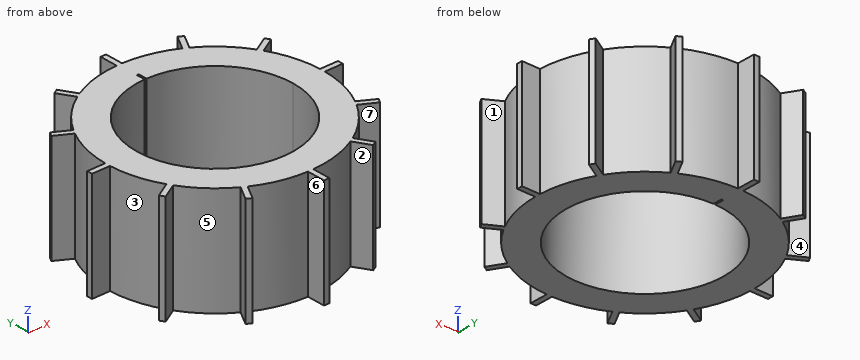
```python
from build123d import *

# Parameters (mm, degrees)
SKETCH1_R           = 60
SKETCH1_R_2         = 43.5
EXTRUSION1_DEPTH    = 60
EXTRUSION3_START    = -60
EXTRUSION3_DEPTH    = 60
BOSS_EXTRUDE2_DEPTH = 60


with BuildPart() as part:
    # Sketch1 → Extrusion1 (new body)
    with BuildSketch(Plane.XY):
        Circle(SKETCH1_R)
        Circle(SKETCH1_R_2, mode=Mode.SUBTRACT)
    extrude(amount=EXTRUSION1_DEPTH)

    # Sketch3 → Extrusion3 (cut)
    with BuildSketch(Plane.XY.offset(60).offset(EXTRUSION3_START)):
        with BuildLine():
            Line((-0.5, 48.5), (-0.5, 43.497126342))
            ThreePointArc((-0.5, 43.497126342), (0, 43.5), (0.5, 43.497126342))
            Line((0.5, 43.497126342), (0.5, 48.5))
            Line((0.5, 48.5), (-0.5, 48.5))
        make_face()
    extrude(amount=EXTRUSION3_DEPTH, mode=Mode.SUBTRACT)

    # Sketch2 → Boss-Extrude2 (add, through all)
    with BuildSketch(Plane.XY.offset(60)):
        with BuildLine():
            Line((33.700961894, 61.371778265), (28.691585429, 52.695283713))
            ThreePointArc((28.691585429, 52.695283713), (30, 51.961524227), (31.28966164, 51.195283713))
            Line((31.28966164, 51.195283713), (36.299038106, 59.871778265))
            Line((36.299038106, 59.871778265), (33.700961894, 61.371778265))
        make_face()
        with BuildLine():
            Line((-1.5, 70), (-1.5, 59.981247069))
            ThreePointArc((-1.5, 59.981247069), (0, 60), (1.5, 59.981247069))
            Line((1.5, 59.981247069), (1.5, 70))
            Line((1.5, 70), (-1.5, 70))
        make_face()
        with BuildLine():
            Line((59.871778265, 36.299038106), (51.195283713, 31.28966164))
            ThreePointArc((51.195283713, 31.28966164), (51.961524227, 30), (52.695283713, 28.691585429))
            Line((52.695283713, 28.691585429), (61.371778265, 33.700961894))
            Line((61.371778265, 33.700961894), (59.871778265, 36.299038106))
        make_face()
        with BuildLine():
            Line((70, 1.5), (59.981247069, 1.5))
            ThreePointArc((59.981247069, 1.5), (60, 0), (59.981247069, -1.5))
            Line((59.981247069, -1.5), (70, -1.5))
            Line((70, -1.5), (70, 1.5))
        make_face()
        with BuildLine():
            Line((61.371778265, -33.700961894), (52.695283713, -28.691585429))
            ThreePointArc((52.695283713, -28.691585429), (51.961524227, -30), (51.195283713, -31.28966164))
            Line((51.195283713, -31.28966164), (59.871778265, -36.299038106))
            Line((59.871778265, -36.299038106), (61.371778265, -33.700961894))
        make_face()
        with BuildLine():
            Line((36.299038106, -59.871778265), (31.28966164, -51.195283713))
            ThreePointArc((31.28966164, -51.195283713), (30, -51.961524227), (28.691585429, -52.695283713))
            Line((28.691585429, -52.695283713), (33.700961894, -61.371778265))
            Line((33.700961894, -61.371778265), (36.299038106, -59.871778265))
        make_face()
        with BuildLine():
            Line((1.5, -70), (1.5, -59.981247069))
            ThreePointArc((1.5, -59.981247069), (0, -60), (-1.5, -59.981247069))
            Line((-1.5, -59.981247069), (-1.5, -70))
            Line((-1.5, -70), (1.5, -70))
        make_face()
        with BuildLine():
            Line((-33.700961894, -61.371778265), (-28.691585429, -52.695283713))
            ThreePointArc((-28.691585429, -52.695283713), (-30, -51.961524227), (-31.28966164, -51.195283713))
            Line((-31.28966164, -51.195283713), (-36.299038106, -59.871778265))
            Line((-36.299038106, -59.871778265), (-33.700961894, -61.371778265))
        make_face()
        with BuildLine():
            Line((-59.871778265, -36.299038106), (-51.195283713, -31.28966164))
            ThreePointArc((-51.195283713, -31.28966164), (-51.961524227, -30), (-52.695283713, -28.691585429))
            Line((-52.695283713, -28.691585429), (-61.371778265, -33.700961894))
            Line((-61.371778265, -33.700961894), (-59.871778265, -36.299038106))
        make_face()
        with BuildLine():
            Line((-70, -1.5), (-59.981247069, -1.5))
            ThreePointArc((-59.981247069, -1.5), (-60, 0), (-59.981247069, 1.5))
            Line((-59.981247069, 1.5), (-70, 1.5))
            Line((-70, 1.5), (-70, -1.5))
        make_face()
        with BuildLine():
            Line((-61.371778265, 33.700961894), (-52.695283713, 28.691585429))
            ThreePointArc((-52.695283713, 28.691585429), (-51.961524227, 30), (-51.195283713, 31.28966164))
            Line((-51.195283713, 31.28966164), (-59.871778265, 36.299038106))
            Line((-59.871778265, 36.299038106), (-61.371778265, 33.700961894))
        make_face()
        with BuildLine():
            Line((-36.299038106, 59.871778265), (-31.28966164, 51.195283713))
            ThreePointArc((-31.28966164, 51.195283713), (-30, 51.961524227), (-28.691585429, 52.695283713))
            Line((-28.691585429, 52.695283713), (-33.700961894, 61.371778265))
            Line((-33.700961894, 61.371778265), (-36.299038106, 59.871778265))
        make_face()
    extrude(amount=-BOSS_EXTRUDE2_DEPTH)


solid = part.part
```
Geometry: final body of the model. Coordinates: model frame, mm. Face numbers are marked on the shaded views. A direction names the side the tool comes from. Coordinates: 2 decimals unless noted, no trailing zeros. Loops run counter-clockwise (first coordinate to the right, second up) from the corner with the lowest first, then second, coordinate; pieces in that order, holes last. Notation, with made-up numbers: (-35, -33) -> (-30, -33) arc R11 ccw to (-30, -20) -> close; hole circle Ø5 at (-15, -30.75). An arc over 180 degrees is marked (long way). Use a Markdown table: item, result. Add a question column.
(1) Line query: line 1 along Y through (x, z) = (0, 18); line 2 along Y through (x, z) = (33, 32); line 3 along X through (y, z) = (0, 31). Output: solid intervals per line, ascending.
(2) Section query A-A, the plane y = 9. Return loops of the section in (x, z).
(3) Pin query (flat end, axial travel): pin 1 Ø1.5 at (y, z) = (46, 17.5) entering from +X; pin 2 Ø12 at (y, z) = (-12, 40) entering from -X; pin 3 Ø3 at (x, z) = (67, 34) entering from -Y; pin 4 Ø10 at (x, y) = (-54.5, 35.5) entering from -Z. Return the tip coordinate at first contact, or that it passes through.
(4) Access query for the marked faces 1, 2, 3 and 4. Directions: +Z, -Z, +X, -X, +Y, -Y. A direction counts if a zero-diameter tool reaches every point of the face in a straight line with its end or side. Return the directions, or none.
(5) Mould query, pull axis Y, two halves, no side actions, for the marked faces 5, 6 and 7. Classes: pulls with the +Y half, pulls with the -Y half, needs draft (parallel to the pull), parting line crosses it, or undercut.
Answer:
| question | item | result |
|---|---|---|
| 1 | line 1 | y = -70 to -43.5, 48.5 to 70 |
| 1 | line 2 | y = -60.16 to -54.16, -50.11 to -28.34, 28.34 to 50.11, 54.16 to 60.16 |
| 1 | line 3 | x = -70 to -43.5, 43.5 to 70 |
| 2 | outline | (-59.32, 0) -> (-42.56, 0) -> (-42.56, 60) -> (-59.32, 60) -> close; (42.56, 0) -> (59.32, 0) -> (59.32, 60) -> (42.56, 60) -> close |
| 3 | pin 1 | stops at x = 39.4 |
| 3 | pin 2 | stops at x = -59.7 |
| 3 | pin 3 | stops at y = -1.5 |
| 3 | pin 4 | stops at z = 0 |
| 4 | face 1 | +Z, -Z, +X |
| 4 | face 2 | +Z, -Z, -Y |
| 4 | face 3 | +Z, -Z, -X |
| 4 | face 4 | +Z, -Z, +Y |
| 5 | face 5 | undercut |
| 5 | face 6 | needs draft |
| 5 | face 7 | pulls with the -Y half |
